Geometry: see drawing. Coordinates: mm, zero at the bounding-box minimum. A direction names the side the tool comes from. Round coordinates to 2 decimals unless told otherwise and drop trailing zeros. Write each loop counter-clockwise with the first axis right and the second up, starting at its lowest first coordinate (ties: lowest second). Pieces come first, ordered by that corner, then holes. Notation, with made-up numbers: M 88,87.25 L 97,87.25 A10 cw 97,106.25 Z; hole C 58,-15 d2. An arc over 180 degrees is marked long. Use one line per item in the form item = value. Start each with the question number.
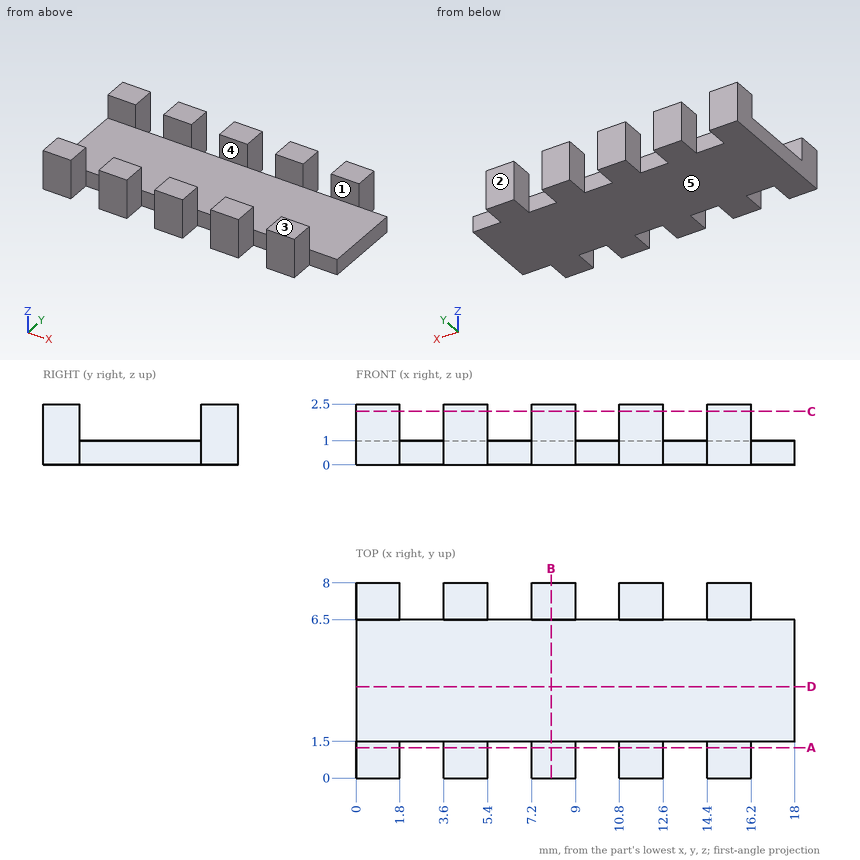
Item 1: Cut plane A-A (y = 1.25). Output: boundary loops of the cut face in (x, z).
Item 2: Ray query, line 1 (X direction, y = 7, z = 0.6); line 2 (Y direction, x = 1.5, z = 2.3); line 3 (Z direction, x = 3, y = 3.5). Return the intervals inside material, ascending. Write a range as from..to.
Item 3: First-contact query: pin 1 (0.5 mm diameter, centred on x = 9.5, z = 0.5, fed in from -Y); pin 2 (1.1 mm diameter, centred on x = 17.5, z = 0.5, fed in from +Y); pin 3 (1.2 mm diameter, centred on y = 7.5, z = 1.5, fed in from +X). Flat tips, straight axial feed; report the tip coordinate or a pass-through.
Item 4: Reachability of the marked faces 4 and 5 from +Z, -Z, +X, -X, +Y, -Y: full face, straight path, thin tool, end or side. Return the list, or none.
Item 5: Cut plane C-C (z = 2.2). Give the number of separate pieces and of enclosed holes in the cut face, plus the area to 3 significant figures.
Item 6: Cut plane B-B (x = 8). Output: boundary loops of the cut face in (y, z), plus the area to 3 significant figures.
Item 7: Draft query along Y for the marked faces 1, 2 and 3. Return one class per face: +Y half, -Y half, draft (parallel to the pull), parting line (faces both ways), or undercut.
Item 8: Cut plane D-D (y = 3.75). Output: boundary loops of the cut face in (x, z).
Final values:
q1.outline = M 0,0 L 1.8,0 L 1.8,2.5 L 0,2.5 Z; M 3.6,0 L 5.4,0 L 5.4,2.5 L 3.6,2.5 Z; M 7.2,0 L 9,0 L 9,2.5 L 7.2,2.5 Z; M 10.8,0 L 12.6,0 L 12.6,2.5 L 10.8,2.5 Z; M 14.4,0 L 16.2,0 L 16.2,2.5 L 14.4,2.5 Z
q2.line_1 = 0..1.8, 3.6..5.4, 7.2..9, 10.8..12.6, 14.4..16.2
q2.line_2 = 0..1.5, 6.5..8
q2.line_3 = 0..1
q3.pin_1 = 1.5
q3.pin_2 = 6.5
q3.pin_3 = 16.2
q4.face_4 = +Z, +X, -X
q4.face_5 = -Z, +X, -X, +Y, -Y
q5.separate_pieces = 10
q5.enclosed_holes = 0
q5.area = 27.0 mm^2
q6.outline = M 0,0 L 8,0 L 8,2.5 L 6.5,2.5 L 6.5,1 L 1.5,1 L 1.5,2.5 L 0,2.5 Z
q6.area = 12.5 mm^2
q7.face_1 = undercut
q7.face_2 = +Y half
q7.face_3 = draft
q8.outline = M 0,0 L 18,0 L 18,1 L 0,1 Z
